```python
from build123d import *

# Parameters (mm, degrees)
F2_R      = 1.85
F2_R_2    = 1
F3_DEPTH  = 3.2
F4_W      = 12
F4_H      = 13.9
F5_DEPTH  = 5
F6_D      = 7
F7_W      = 2
F7_H      = 1
F8_DEPTH  = 6
F9_W      = 7
F9_H      = 10
F10_DEPTH = 5
F11_DEPTH = 3.2
F13_DEPTH = 1.5
F14_DEPTH = 25
F15_R     = 5
F16_DEPTH = 0.5
F17_W     = 2
F17_H     = 2
F18_DEPTH = 5.1


with BuildPart() as f1:
    # F0 (on Top) → F1 (revolve)
    with BuildSketch(Plane.XY):
        Polygon((-9.3, -5.1), (0, -5.1), (0, 3.2), (-9.9, 3.2), (-9.9, 0), (-9.3, 0), align=None)
    revolve(axis=Axis((0, -0.95, 0), (0, -1, 0)))

    # F4 (on face) → F5 (cut)
    with BuildSketch(Plane.XZ.offset(5.1)):
        Rectangle(F4_W, F4_H)
    extrude(amount=-F5_DEPTH, mode=Mode.SUBTRACT)

    # F6 (through all)
    with Locations(Plane.XZ.offset(5.1)):
        with Locations((0, 0)):
            Hole(F6_D / 2)

    # F7 (on face) → F8 (cut)
    with BuildSketch(Plane.XZ.offset(5.1)):
        with Locations((0, 6.45)):
            Rectangle(F7_W, F7_H)
    extrude(amount=-F8_DEPTH, mode=Mode.SUBTRACT)

    # F9 (on face) → F10 (cut)
    with BuildSketch(Plane.XZ.offset(5.1)):
        with Locations((0, 11.95)):
            Rectangle(F9_W, F9_H)
    extrude(amount=-F10_DEPTH, mode=Mode.SUBTRACT)


with BuildPart() as f3:
    # F2 (on face) → F3 (new body)
    with BuildSketch(Plane(origin=(0, 3.2, 0), x_dir=(-1, 0, 0), z_dir=(0, 1, 0))):
        with BuildLine():
            Line((-11.75, -2.7), (-9.5247047198, -2.7))
            ThreePointArc((-9.5247047198, -2.7), (-9.8057273245, -1.3629789569), (-9.9, 0))
            ThreePointArc((-9.9, 0), (-9.8057273245, 1.3629789569), (-9.5247047198, 2.7))
            Line((-9.5247047198, 2.7), (-11.75, 2.7))
            ThreePointArc((-11.75, 2.7), (-13.6591883092, 1.9091883092), (-14.45, 0))
            ThreePointArc((-14.45, 0), (-13.6591883092, -1.9091883092), (-11.75, -2.7))
        make_face()
        with Locations((-11.75, 0)):
            Circle(F2_R, mode=Mode.SUBTRACT)
        with Locations((-11.75, 0)):
            Circle(F2_R)
        with Locations((-11.75, 0)):
            Circle(F2_R_2, mode=Mode.SUBTRACT)
    extrude(amount=-F3_DEPTH)


with BuildPart() as f11:
    # F2 (on face) → F11 (new body)
    with BuildSketch(Plane(origin=(0, 3.2, 0), x_dir=(-1, 0, 0), z_dir=(0, 1, 0))):
        with BuildLine():
            ThreePointArc((9.9, 0), (9.8057273245, -1.3629789569), (9.5247047198, -2.7))
            Line((9.5247047198, -2.7), (11.75, -2.7))
            ThreePointArc((11.75, -2.7), (13.6591883092, -1.9091883092), (14.45, 0))
            ThreePointArc((14.45, 0), (13.6591883092, 1.9091883092), (11.75, 2.7))
            Line((11.75, 2.7), (9.5247047198, 2.7))
            ThreePointArc((9.5247047198, 2.7), (9.8057273245, 1.3629789569), (9.9, 0))
        make_face()
        with BuildLine():
            ThreePointArc((13.6, 0), (11.75, -1.85), (9.9, 0))
            ThreePointArc((9.9, 0), (11.75, 1.85), (13.6, 0))
        make_face(mode=Mode.SUBTRACT)
        with BuildLine():
            ThreePointArc((13.6, 0), (11.75, 1.85), (9.9, 0))
            ThreePointArc((9.9, 0), (11.75, -1.85), (13.6, 0))
        make_face()
        with Locations((11.75, 0)):
            Circle(F2_R_2, mode=Mode.SUBTRACT)
        with Locations((11.75, 0)):
            Circle(F2_R_2)
    extrude(amount=-F11_DEPTH)


with BuildPart() as f3_1:
    add(f3.part)

    # F12: union F11, F1
    add(f11.part)
    add(f1.part)

    # F2 (on face) → F13 (cut)
    with BuildSketch(Plane(origin=(0, 3.2, 0), x_dir=(-1, 0, 0), z_dir=(0, 1, 0))):
        with BuildLine():
            ThreePointArc((13.6, 0), (11.75, 1.85), (9.9, 0))
            ThreePointArc((9.9, 0), (11.75, -1.85), (13.6, 0))
        make_face()
        with Locations((11.75, 0)):
            Circle(F2_R_2, mode=Mode.SUBTRACT)
        with Locations((-11.75, 0)):
            Circle(F2_R)
        with Locations((-11.75, 0)):
            Circle(F2_R_2, mode=Mode.SUBTRACT)
    extrude(amount=-F13_DEPTH, mode=Mode.SUBTRACT)

    # F2 (on face) → F14 (cut)
    with BuildSketch(Plane(origin=(0, 3.2, 0), x_dir=(-1, 0, 0), z_dir=(0, 1, 0))):
        with Locations((11.75, 0)):
            Circle(F2_R_2)
    extrude(amount=-F14_DEPTH, mode=Mode.SUBTRACT)

    # F15 (on face) → F16 (cut)
    with BuildSketch(Plane.XZ.offset(0.1)):
        Circle(F15_R)
    extrude(amount=-F16_DEPTH, mode=Mode.SUBTRACT)

    # F17 (on face) → F18 (cut, through all)
    with BuildSketch(Plane.XZ.offset(5.1)):
        with Locations((-6, -6.95)):
            Rectangle(F17_W, F17_H)
        with Locations((6, -6.95)):
            Rectangle(F17_W, F17_H)
    extrude(amount=-F18_DEPTH, mode=Mode.SUBTRACT)


solid = f3_1.part
```
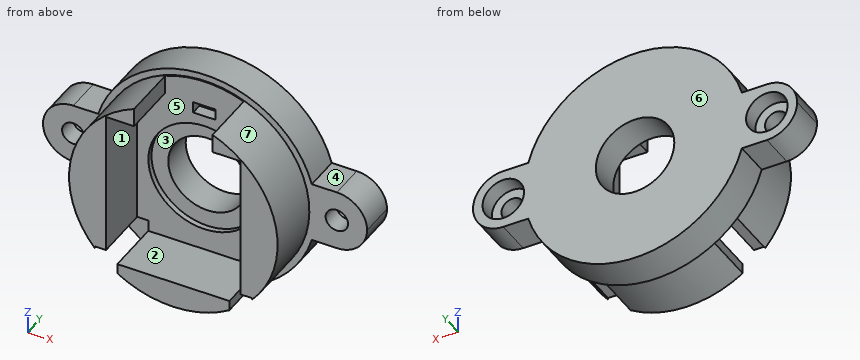
The listing builds one solid part. Answer for the finished solid, in the listing's coordinates (mm). Face numbers are marked on the shaded views. A direction names the side the tool comes from. Round coordinates to 2 decimals unless told otherwise and drop trailing zeros. Loops run counter-clockwise (first coordinate to the right, second up) from the corner with the lowest first, then second, coordinate; pieces in that order, holes last. Notation, with made-up numbers: (-27.5, 16.25) - (-9.5, 16.25) arc R27 ccw to (-9.5, 48.25) - close; hole circle Ø3 at (-21.5, 2.5). An arc over 180 degrees is marked (long way). Use one line per item in the form item = value. Start each with the question number.
1. The part is cut by section D-D on y = 1.25. Determine the outline of the cut face in (x, z).
2. The part is cut by section A-A on x = 0. Determine the outline of the cut face in (y, z).
3. The part is cut by section B-B on y = -3.25. Determine the outline of the cut face in (x, z), then the cut area to 3 significant figures.
4. For a pull along Z with two mould halves and no side action, classify the marked faces 5, 6 and 7 as pulls with the +Z half, pulls with the -Z half, needs draft (parallel to the pull), parting line crosses it, or undercut.
5. The part is cut by section C-C on z = 1.5. Determine the outline of the cut face in (x, y) (3 decimals).
6. Given pin 1 Ø1.5 at (y, z) = (-2, -7) entering from +X; pin 2 Ø3 at (x, y) = (-3.5, 0.5) entering from +Z; pin 3 Ø0.8 at (x, z) = (0, 6) entering from -Y, each flat-ended and moving along its own axis, determine where each tip first touches the part or whether it passes through.
7. Consider line 1 (Z direction, x = 0, y = 0.05); line 2 (Z direction, x = 11.75, y = 0.95); line 3 (Z direction, x = -11.75, y = 2.75). Determine where each line is inside the solid, lowest interval first. Write a range as [from, to].
8. A tool of negligible diameter and unlimited length cuts with its end or side. For the marked faces 1, 2, 3 and 4, from which of +Z, -Z, +X, -X, +Y, -Y can it reach the whole face along a straight path? Write none if from no direction.
Geometry check:
q1.outline = (-11.75, -2.7) - (-9.52, -2.7) arc R9.9 ccw to (9.52, -2.7) - (11.75, -2.7) arc R2.7 ccw to (11.75, 2.7) - (9.52, 2.7) arc R9.9 ccw to (-9.52, 2.7) - (-11.75, 2.7) arc R2.7 ccw to start; hole circle Ø2 at (-11.75, 0); hole circle Ø7 at (0, 0); hole circle Ø2 at (11.75, 0)
q2.outline = (-5.1, -9.3) - (0, -9.3) - (0, -9.9) - (3.2, -9.9) - (3.2, -3.5) - (0.4, -3.5) - (0.4, -5) - (-0.1, -5) - (-0.1, -6.95) - (-5.1, -6.95) - close; (-0.1, 5) - (0.4, 5) - (0.4, 3.5) - (3.2, 3.5) - (3.2, 9.9) - (0, 9.9) - (0, 9.3) - (-0.1, 9.3) - (-0.1, 6.95) - (0.9, 6.95) - (0.9, 5.95) - (-0.1, 5.95) - close
q3.outline = (-7, -6.12) - (-7, -5.95) - (-6, -5.95) - (-6, 6.95) - (-3.5, 6.95) - (-3.5, 8.62) arc R9.3 ccw to start; (-5, -7.84) arc R9.3 ccw to (5, -7.84) - (5, -6.95) - (-5, -6.95) - close; (3.5, 6.95) - (6, 6.95) - (6, -5.95) - (7, -5.95) - (7, -6.12) arc R9.3 ccw to (3.5, 8.62) - close
q3.area = 87.6 mm^2
q4.face_5 = undercut
q4.face_6 = needs draft
q4.face_7 = parting line crosses it
q5.outline = (-13.995, 0) - (-9.178, 0) - (-9.178, -5.1) - (-6, -5.1) - (-6, -0.1) - (-4.77, -0.1) - (-4.77, 0.4) - (-3.162, 0.4) - (-3.162, 3.2) - (-10.667, 3.2) - (-10.667, 1.7) - (-12.833, 1.7) - (-12.833, 3.2) - (-13.995, 3.2) - close; (3.162, 0.4) - (4.77, 0.4) - (4.77, -0.1) - (6, -0.1) - (6, -5.1) - (9.178, -5.1) - (9.178, 0) - (13.995, 0) - (13.995, 3.2) - (12.833, 3.2) - (12.833, 1.7) - (10.667, 1.7) - (10.667, 3.2) - (3.162, 3.2) - close
q6.pin_1 = 5
q6.pin_2 = 9.7
q6.pin_3 = -0.1
q7.line_1 = [-9.9, -5], [5, 5.95], [6.95, 9.9]
q7.line_2 = [-2.7, -1], [1, 2.7]
q7.line_3 = [-2.7, -1.85], [1.85, 2.7]
q8.face_1 = -Z, -Y
q8.face_2 = +X, -X, -Y
q8.face_3 = -Y
q8.face_4 = +Z, +X, +Y, -Y
